Design review of the part built by this model. Coordinates are the model's own, in mm. Round coordinates to 2 decimals unless told otherwise and drop trailing zeros. Loops run counter-clockwise (first coordinate to the right, second up) from the corner with the lowest first, then second, coordinate; pieces in that order, holes last. Notation, with made-up numbers: (22, 59.5) -> (29, 59.5) arc R34 ccw to (29, 98.5) -> close; hole circle Ø2 at (43, -2). An arc over 180 degrees is marked (long way). Use a Markdown table: item, result. Add a question column.
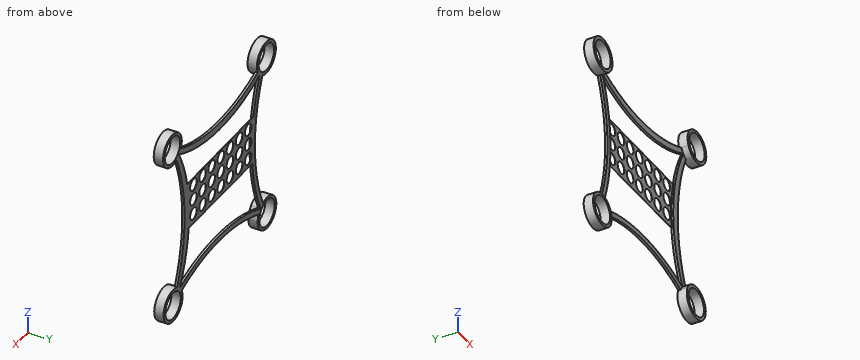
from build123d import *

# Parameters (mm, degrees)
F0_R     = 36.5947560904
F0_R_2   = 36.5964348683
F1_DEPTH = 6.35
F2_DEPTH = 25.4
F0_R_3   = 16.0861270077
F4_DEPTH = 0.762


with BuildPart() as f1:
    # F0 (on Front) → F1 (new body)
    with BuildSketch(Plane.XZ):
        with BuildLine():
            ThreePointArc((188.5982540505, 184.8449959839), (6.2169992483, 146.7538533434), (-176.8098994137, 181.6108700985))
            ThreePointArc((-176.8098994137, 181.6108700985), (-180.7223168449, 174.7262392004), (-185.7909638385, 168.6423284177))
            ThreePointArc((-185.7909638385, 168.6423284177), (6.1536082496, 128.2088675402), (197.1884370844, 172.7428734756))
            ThreePointArc((197.1884370844, 172.7428734756), (192.3851525579, 178.4332152803), (188.5982540505, 184.8449959839))
        make_face()
        with BuildLine():
            ThreePointArc((-189.4134185263, -217.1728797195), (-184.6334375627, -222.8381994872), (-180.8650399113, -229.2212430576))
            ThreePointArc((-180.8650399113, -229.2212430577), (1.5143996628, -191.1214074538), (184.542960009, -225.969700813))
            ThreePointArc((184.542960009, -225.969700813), (188.4782832358, -219.102761645), (193.5517747378, -213.0281170945))
            ThreePointArc((193.5517747378, -213.0281170945), (1.6628304665, -177.5550425479), (-189.4134185263, -217.1728797195))
        make_face()
        with BuildLine():
            ThreePointArc((-185.7909638385, 168.6423284177), (-180.7223168449, 174.7262392004), (-176.8098994137, 181.6108700985))
            ThreePointArc((-176.8098994137, 181.6108700985), (-185.818640213, 168.6699018858), (-198.7259600139, 159.613016956))
            ThreePointArc((-198.7259600139, 159.613016956), (-191.8559511005, 163.5510533052), (-185.7909638385, 168.6423284177))
        make_face()
        with BuildLine():
            ThreePointArc((209.2824572603, 164.1388911845), (197.1933772998, 172.7468130702), (188.5982540505, 184.8449959839))
            ThreePointArc((188.5982540505, 184.8449959839), (192.3851525579, 178.4332152803), (197.1884370844, 172.7428734756))
            ThreePointArc((197.1884370844, 172.7428734756), (202.8741139753, 167.9329813574), (209.2824572603, 164.1388911845))
        make_face()
        with BuildLine():
            ThreePointArc((-189.4134185263, -217.1728797195), (-189.4317221538, -217.1805770734), (-189.4500254799, -217.1882751439))
            ThreePointArc((-189.4500254799, -217.1882751439), (-184.6593067493, -222.8492971242), (-180.8650399113, -229.2212430576))
            ThreePointArc((-180.8650399113, -229.2212430576), (-184.6334375627, -222.8381994872), (-189.4134185263, -217.1728797195))
        make_face()
        with BuildLine():
            ThreePointArc((-189.4343998959, -217.1518790975), (-195.0954466485, -212.3666234088), (-201.4751684195, -208.5923324203))
            ThreePointArc((-201.4751684195, -208.5923324203), (-195.1066812913, -212.3924018294), (-189.4500254799, -217.1882751439))
            ThreePointArc((-189.4500254799, -217.1882751439), (-189.4422123275, -217.1700772754), (-189.4343998959, -217.1518790975))
        make_face()
        with BuildLine():
            ThreePointArc((193.5611194533, -213.0318108647), (199.6168571715, -207.9342533355), (206.4672712931, -203.9682883284))
            ThreePointArc((206.4672712931, -203.9682883284), (199.6138346269, -207.9279426554), (193.5567810212, -213.0230931091))
            ThreePointArc((193.5567810212, -213.0230931091), (193.5589502123, -213.0274519993), (193.5611194533, -213.0318108647))
        make_face()
        with BuildLine():
            ThreePointArc((184.542960009, -225.969700813), (188.4848520946, -219.1054063219), (193.5611194533, -213.0318108647))
            ThreePointArc((193.5611194533, -213.0318108647), (193.5564471047, -213.0299639564), (193.5517747378, -213.0281170945))
            ThreePointArc((193.5517747378, -213.0281170945), (188.4782832358, -219.102761645), (184.542960009, -225.969700813))
        make_face()
        with BuildLine():
            ThreePointArc((209.2824572603, 164.1388911845), (202.8741139753, 167.9329813574), (197.1884370844, 172.7428734756))
            ThreePointArc((197.1884370844, 172.7428734756), (173.8608394568, 119.3607598746), (158.0536671707, 63.2897319912))
            ThreePointArc((158.0536671707, 63.2897319912), (149.6447133976, -1.2966260467), (151.2048073719, -66.4094070881))
            ThreePointArc((151.2048073719, -66.4094070881), (165.7451521785, -141.6330734425), (193.5567810212, -213.0230931091))
            ThreePointArc((193.5567810212, -213.0230931091), (199.6138346269, -207.9279426554), (206.4672712931, -203.9682883284))
            ThreePointArc((206.4672712931, -203.9682883284), (170.9071745934, -19.6319794971), (209.2824572603, 164.1388911845))
        make_face()
        with BuildLine():
            ThreePointArc((-185.7909638385, 168.6423284177), (-191.8559511005, 163.5510533052), (-198.7259600139, 159.613016956))
            ThreePointArc((-198.7259600139, 159.613016956), (-163.1149600765, -24.7658110633), (-201.4751684195, -208.5923324203))
            ThreePointArc((-201.4751684195, -208.5923324203), (-195.0954466485, -212.3666234088), (-189.4343998959, -217.1518790975))
            ThreePointArc((-189.4343998959, -217.1518790975), (-164.1007583774, -142.312832824), (-150.8712536248, -64.417669664))
            ThreePointArc((-150.8712536248, -64.417669664), (-149.3480842089, 1.6053439773), (-156.5386111016, 67.2533043292))
            ThreePointArc((-156.5386111016, 67.2533043292), (-168.4828359414, 118.721602223), (-185.7909638385, 168.6423284177))
        make_face()
        with BuildLine():
            ThreePointArc((-198.7259600139, 159.613016956), (-185.818640213, 168.6699018858), (-176.8098994137, 181.6108700985))
            ThreePointArc((-176.8098994137, 181.6108700985), (-173.6989412825, 190.8575184286), (-172.6455822149, 200.5564359203))
            ThreePointArc((-172.6455822149, 200.5564359203), (-255.9288759313, 224.828589011), (-198.7259600139, 159.613016956))
        make_face()
        with Locations((-217.8241774175, 200.5564359203)):
            Circle(F0_R, mode=Mode.SUBTRACT)
        with BuildLine():
            ThreePointArc((273.1536156326, 204.1844323112), (218.7448667821, 247.5538425266), (188.5982540505, 184.8449959839))
            ThreePointArc((188.5982540505, 184.8449959839), (197.1933772998, 172.7468130702), (209.2824572603, 164.1388911845))
            ThreePointArc((209.2824572603, 164.1388911845), (252.2970589417, 166.4910302494), (273.1536156326, 204.1844323112))
        make_face()
        with Locations((228.6642844479, 204.1844323112)):
            Circle(F0_R_2, mode=Mode.SUBTRACT)
        with BuildLine():
            ThreePointArc((270.7215789425, -244.9095990816), (249.8240085798, -206.8149571431), (206.4672712931, -203.9682883284))
            ThreePointArc((206.4672712931, -203.9682883284), (199.6168571715, -207.9342533355), (193.5611194533, -213.0318108647))
            ThreePointArc((193.5611194533, -213.0318108647), (188.4848520946, -219.1054063219), (184.542960009, -225.969700813))
            ThreePointArc((184.542960009, -225.969700813), (215.8550559689, -289.0272659162), (270.7215789425, -244.9095990816))
        make_face()
        with Locations((225.5510122517, -244.9095990816)):
            Circle(F0_R_2, mode=Mode.SUBTRACT)
        with BuildLine():
            ThreePointArc((-189.4500254799, -217.1882751439), (-195.1066812913, -212.3924018294), (-201.4751684195, -208.5923324203))
            ThreePointArc((-201.4751684195, -208.5923324203), (-258.2891293584, -272.0079714896), (-176.4637429727, -248.4712856786))
            ThreePointArc((-176.4637429727, -248.4712856786), (-177.5780831864, -238.5978926999), (-180.8650399113, -229.2212430576))
            ThreePointArc((-180.8650399113, -229.2212430576), (-184.6593067493, -222.8492971242), (-189.4500254799, -217.1882751439))
        make_face()
        with Locations((-220.7615444029, -248.4712856786)):
            Circle(F0_R_2, mode=Mode.SUBTRACT)
    extrude(amount=F1_DEPTH)

    # F0 (on Front) → F2 (join)
    with BuildSketch(Plane.XZ):
        with BuildLine():
            ThreePointArc((-189.4500254799, -217.1882751439), (-195.1066812913, -212.3924018294), (-201.4751684195, -208.5923324203))
            ThreePointArc((-201.4751684195, -208.5923324203), (-258.2891293584, -272.0079714896), (-176.4637429727, -248.4712856786))
            ThreePointArc((-176.4637429727, -248.4712856786), (-177.5780831864, -238.5978926999), (-180.8650399113, -229.2212430576))
            ThreePointArc((-180.8650399113, -229.2212430576), (-184.6593067493, -222.8492971242), (-189.4500254799, -217.1882751439))
        make_face()
        with Locations((-220.7615444029, -248.4712856786)):
            Circle(F0_R_2, mode=Mode.SUBTRACT)
        with BuildLine():
            ThreePointArc((270.7215789425, -244.9095990816), (249.8240085798, -206.8149571431), (206.4672712931, -203.9682883284))
            ThreePointArc((206.4672712931, -203.9682883284), (199.6168571715, -207.9342533355), (193.5611194533, -213.0318108647))
            ThreePointArc((193.5611194533, -213.0318108647), (188.4848520946, -219.1054063219), (184.542960009, -225.969700813))
            ThreePointArc((184.542960009, -225.969700813), (215.8550559689, -289.0272659162), (270.7215789425, -244.9095990816))
        make_face()
        with Locations((225.5510122517, -244.9095990816)):
            Circle(F0_R_2, mode=Mode.SUBTRACT)
        with BuildLine():
            ThreePointArc((273.1536156326, 204.1844323112), (218.7448667821, 247.5538425266), (188.5982540505, 184.8449959839))
            ThreePointArc((188.5982540505, 184.8449959839), (197.1933772998, 172.7468130702), (209.2824572603, 164.1388911845))
            ThreePointArc((209.2824572603, 164.1388911845), (252.2970589417, 166.4910302494), (273.1536156326, 204.1844323112))
        make_face()
        with Locations((228.6642844479, 204.1844323112)):
            Circle(F0_R_2, mode=Mode.SUBTRACT)
        with BuildLine():
            ThreePointArc((-198.7259600139, 159.613016956), (-185.818640213, 168.6699018858), (-176.8098994137, 181.6108700985))
            ThreePointArc((-176.8098994137, 181.6108700985), (-173.6989412825, 190.8575184286), (-172.6455822149, 200.5564359203))
            ThreePointArc((-172.6455822149, 200.5564359203), (-255.9288759313, 224.828589011), (-198.7259600139, 159.613016956))
        make_face()
        with Locations((-217.8241774175, 200.5564359203)):
            Circle(F0_R, mode=Mode.SUBTRACT)
    extrude(amount=F2_DEPTH)

    # F0 (on Front) → F4 (join)
    with BuildSketch(Plane.XZ):
        with BuildLine():
            ThreePointArc((158.0536671707, 63.2897319912), (0.7607458029, 65.5269153094), (-156.5386111016, 67.2533043292))
            ThreePointArc((-156.5386111016, 67.2533043292), (-149.3480842089, 1.6053439773), (-150.8712536248, -64.417669664))
            ThreePointArc((-150.8712536248, -64.417669664), (0.1662637574, -65.4913599309), (151.2048073719, -66.4094070881))
            ThreePointArc((151.2048073719, -66.4094070881), (149.6447133976, -1.2966260467), (158.0536671707, 63.2897319912))
        make_face()
        with Locations((-132.0719718933, -38.919291311)):
            Circle(F0_R_3, mode=Mode.SUBTRACT)
        with Locations((-88.6379718933, -38.919291311)):
            Circle(F0_R_3, mode=Mode.SUBTRACT)
        with Locations((-45.2039718933, -38.919291311)):
            Circle(F0_R_3, mode=Mode.SUBTRACT)
        with Locations((-1.7699718933, -38.919291311)):
            Circle(F0_R_3, mode=Mode.SUBTRACT)
        with Locations((41.6640281067, -38.919291311)):
            Circle(F0_R_3, mode=Mode.SUBTRACT)
        with Locations((85.0980281067, -38.919291311)):
            Circle(F0_R_3, mode=Mode.SUBTRACT)
        with Locations((128.5320281067, -38.919291311)):
            Circle(F0_R_3, mode=Mode.SUBTRACT)
        with Locations((-132.0719718933, 2.736708689)):
            Circle(F0_R_3, mode=Mode.SUBTRACT)
        with Locations((-132.0719718933, 44.392708689)):
            Circle(F0_R_3, mode=Mode.SUBTRACT)
        with Locations((-88.6379718933, 2.736708689)):
            Circle(F0_R_3, mode=Mode.SUBTRACT)
        with Locations((-88.6379718933, 44.392708689)):
            Circle(F0_R_3, mode=Mode.SUBTRACT)
        with Locations((-45.2039718933, 2.736708689)):
            Circle(F0_R_3, mode=Mode.SUBTRACT)
        with Locations((-1.7699718933, 2.736708689)):
            Circle(F0_R_3, mode=Mode.SUBTRACT)
        with Locations((-45.2039718933, 44.392708689)):
            Circle(F0_R_3, mode=Mode.SUBTRACT)
        with Locations((-1.7699718933, 44.392708689)):
            Circle(F0_R_3, mode=Mode.SUBTRACT)
        with Locations((41.6640281067, 2.736708689)):
            Circle(F0_R_3, mode=Mode.SUBTRACT)
        with Locations((41.6640281067, 44.392708689)):
            Circle(F0_R_3, mode=Mode.SUBTRACT)
        with Locations((85.0980281067, 2.736708689)):
            Circle(F0_R_3, mode=Mode.SUBTRACT)
        with Locations((128.5320281067, 2.736708689)):
            Circle(F0_R_3, mode=Mode.SUBTRACT)
        with Locations((85.0980281067, 44.392708689)):
            Circle(F0_R_3, mode=Mode.SUBTRACT)
        with Locations((128.5320281067, 44.392708689)):
            Circle(F0_R_3, mode=Mode.SUBTRACT)
    extrude(amount=F4_DEPTH)


solid = f1.part
1. Consider section D-D on x = 90. State the section outline as (y, z) points, plus the area to 3 significant figures.
2. Consider section C-C on x = 228. State the section outline as (y, z) points.
3. Consider section B-B on z = -120. State the section outline as (x, y) points.
4. To check wall thickness, follow probe 1 along X at (y, z) = (-4.25, -242); probe 2 along X at (y, z) = (-14.75, -268.5); probe 3 along Z at (x, y) = (209.5, -12.75). State the ranges of each line that lie inside material, in increasing order. Write a range as from..to.
5. Insertion check: P1, Ø10, axis at x = -211, z = -196.5, coming from the -Y side. The pin has a flat end and moves straight along its axis. Give the tip position at first contact, or say it passes through.
Verdict:
| question | item | result |
|---|---|---|
| 1 | outline | (-6.35, -198.62) -> (0, -198.62) -> (0, -184.34) -> (-6.35, -184.34) -> close; (-6.35, 136.95) -> (0, 136.95) -> (0, 154.94) -> (-6.35, 154.94) -> close; (-0.76, -66.06) -> (0, -66.06) -> (0, -54.24) -> (-0.76, -54.24) -> close; (-0.76, -23.6) -> (0, -23.6) -> (0, -12.58) -> (-0.76, -12.58) -> close; (-0.76, 18.06) -> (0, 18.06) -> (0, 29.07) -> (-0.76, 29.07) -> close; (-0.76, 59.71) -> (0, 59.71) -> (0, 64.32) -> (-0.76, 64.32) -> close |
| 1 | area | 234 mm² |
| 2 | outline | (-25.4, -290.01) -> (0, -290.01) -> (0, -281.42) -> (-25.4, -281.42) -> close; (-25.4, -208.4) -> (0, -208.4) -> (0, -199.81) -> (-25.4, -199.81) -> close; (-25.4, 159.7) -> (0, 159.7) -> (0, 167.59) -> (-25.4, 167.59) -> close; (-25.4, 240.77) -> (0, 240.77) -> (0, 248.67) -> (-25.4, 248.67) -> close |
| 3 | outline | (-173.45, -6.35) -> (-159.01, -6.35) -> (-159.01, 0) -> (-173.45, 0) -> close; (160.11, -6.35) -> (180.81, -6.35) -> (180.81, 0) -> (160.11, 0) -> close |
| 4 | probe 1 | x = -264.58..-256.78, -184.74..-176.94, 180.47..189.07, 262.03..270.63 |
| 4 | probe 2 | x = -260.27..-251.39, -190.13..-181.25, 187.03..197.57, 253.53..264.07 |
| 4 | probe 3 | z = -287.13..-277.8, -212.02..-202.69, 164.03..173.01, 235.36..244.33 |
| 5 | P1 | passes through |
